from build123d import *

# Parameters (mm, degrees)
EXTRUDE_1_DEPTH        = 900
EXTRUDE_1_2_DEPTH      = 900
EXTRUDE_2_DEPTH        = 1720
EXTRUDE_2_2_DEPTH      = 1720
SKETCH_4_W             = 50
SKETCH_4_H             = 60
CUT_EXTRUDE_1_DEPTH    = 10
SKETCH_5_W             = 50
SKETCH_5_H             = 60
CUT_EXTRUDE_2_DEPTH    = 10
SKETCH_6_W             = 60
SKETCH_6_H             = 25
EXTRUDE_3_DEPTH        = 1720
PATTERN_LINEAR_1_COUNT = 2
PATTERN_LINEAR_1_PITCH = 600
SKETCH_7_W             = 25
SKETCH_7_H             = 60
EXTRUDE_4_DEPTH        = 1729
PATTERN_LINEAR_2_COUNT = 5
PATTERN_LINEAR_2_PITCH = 300


with BuildPart() as part:
    # Sketch 1 → Extrude 1 (new, symmetric)
    with BuildSketch(Plane(origin=(0, 0, 0), x_dir=(0, 0, -1), z_dir=(1, 0, 0))):
        Polygon((30, 0), (-30, 0), (-30, 40), (-10, 40), (-10, 50), (10, 50), (10, 40), (30, 40), align=None)
    extrude(amount=EXTRUDE_1_DEPTH, both=True)

    # Sketch 5 → Cut-Extrude 2 (cut)
    with BuildSketch(Plane(origin=(0, 40, 0), x_dir=(1, 0, 0), z_dir=(0, 1, 0))):
        with Locations((-875, 0)):
            Rectangle(SKETCH_5_W, SKETCH_5_H)
        with Locations((875, 0)):
            Rectangle(SKETCH_5_W, SKETCH_5_H)
    extrude(amount=CUT_EXTRUDE_2_DEPTH, mode=Mode.SUBTRACT)



with BuildPart() as body_2:
    # Sketch 1 → Extrude 1 2 (new, symmetric)
    with BuildSketch(Plane(origin=(0, 0, 0), x_dir=(0, 0, -1), z_dir=(1, 0, 0))):
        Polygon((30, 1800), (30, 1760), (10, 1760), (10, 1750), (-10, 1750), (-10, 1760), (-30, 1760), (-30, 1800), align=None)
    extrude(amount=EXTRUDE_1_2_DEPTH, both=True)

    # Sketch 4 → Cut-Extrude 1 (cut)
    with BuildSketch(Plane.XZ.offset(-1760)):
        with Locations((-875, 0)):
            Rectangle(SKETCH_4_W, SKETCH_4_H)
        with Locations((875, 0)):
            Rectangle(SKETCH_4_W, SKETCH_4_H)
    extrude(amount=CUT_EXTRUDE_1_DEPTH, mode=Mode.SUBTRACT)


with BuildPart() as body_3:
    # Sketch 3 → Extrude 2 (new body)
    with BuildSketch(Plane.XZ.offset(-1760)):
        Polygon((-900, -30), (-900, 30), (-860, 30), (-860, 10), (-850, 10), (-850, -10), (-860, -10), (-860, -30), align=None)
    extrude(amount=EXTRUDE_2_DEPTH)



with BuildPart() as body_4:
    # Sketch 3 → Extrude 2 2 (new body)
    with BuildSketch(Plane.XZ.offset(-1760)):
        Polygon((860, -30), (900, -30), (900, 30), (860, 30), (860, 10), (850, 10), (850, -10), (860, -10), align=None)
    extrude(amount=EXTRUDE_2_2_DEPTH)


with BuildPart() as body_3_1:
    add(body_3.part)

    add(body_4.part)  # Extrude 3 merges body 4
    # Sketch 6 → Extrude 3 (add)
    with BuildSketch(Plane.ZY.offset(-860)):
        with Locations((0, 1200)):
            Rectangle(SKETCH_6_W, SKETCH_6_H)
    extrude_3 = extrude(amount=EXTRUDE_3_DEPTH)

    # Pattern Linear 1: Extrude 3 ×2
    with Locations(*[(0, -i * PATTERN_LINEAR_1_PITCH, 0) for i in range(1, PATTERN_LINEAR_1_COUNT)]):
        add(extrude_3)


with BuildPart() as part_1:
    add(part.part)

    add(body_2.part)  # Extrude 4 merges body 2

    add(body_3_1.part)  # Extrude 4 merges body 3
    # Sketch 7 → Extrude 4 (add)
    with BuildSketch(Plane.XZ.offset(-1760)):
        with Locations((-600, 0)):
            Rectangle(SKETCH_7_W, SKETCH_7_H)
    extrude_4 = extrude(amount=EXTRUDE_4_DEPTH)

    # Pattern Linear 2: Extrude 4 ×5
    with Locations(*[(i * PATTERN_LINEAR_2_PITCH, 0, 0) for i in range(1, PATTERN_LINEAR_2_COUNT)]):
        add(extrude_4)


solid = part_1.part
The model under review builds one solid part; all positions refer to its coordinate system, in mm. A direction names the side the tool comes from. Round coordinates to 2 decimals unless told otherwise and drop trailing zeros. Loops run counter-clockwise (first coordinate to the right, second up) from the corner with the lowest first, then second, coordinate; pieces in that order, holes last. Notation, with made-up numbers: (57.25, 8) -> (62.25, 8) arc R22 cw to (62.25, 34) -> close; hole circle Ø8 at (25.5, -11). An arc over 180 degrees is marked (long way). One line per question, with ' | ' between items. Start each with the question number.
Item 1: Wall thickness on line 1 along Y through (x, z) = (348, 5); line 2 along Y through (x, z) = (-767.5, 18.5): over which ranges is each line inside the solid? List them lowest first. Write a range as [from, to].
Item 2: Machinability: for faces 1 (the face through (855, 315, -10)), 2 (the face through (-448, 612.5, 0)), 3 (the face through (-855, 315, 10)), which of the approach directions +Z, -Z, +X, -X, +Y, -Y give a long, thin tool a straight path to every point of the face, cutting with its end or side? Answer none if there is none.
Item 3: Add section A-A, the plane x = 192.5. Write out the cut boundary in (y, z).
Item 4: Add section B-B, the plane y = 1316. Count the separate pieces of the cut face and the enclosed holes in it, then the cut area to 3 significant figures.
Item 5: For pin 1 (3 mm diameter, centred on x = -159.5, y = 42.5, fed in from -Z), flat-tipped, find the tip position at first contact; note if it passes through.
Item 6: Draft analysis for pull direction Y (two halves, no side actions). For faces 4 (the face through (13, 0, 0)), 5 (the face through (152, 587.5, 0)), state which applies: +Y half, -Y half, draft (parallel to the pull), parting line (faces both ways), or undercut.
Return value:
1) line 1: y = [0, 50], [587.5, 612.5], [1187.5, 1212.5], [1750, 1800] | line 2: y = [0, 40], [587.5, 612.5], [1187.5, 1212.5], [1760, 1800]
2) face 1: -Z | face 2: +Z, -Z | face 3: +Z
3) outline: (0, -30) -> (40, -30) -> (40, -10) -> (50, -10) -> (50, 10) -> (40, 10) -> (40, 30) -> (0, 30) -> close; (587.5, -30) -> (612.5, -30) -> (612.5, 30) -> (587.5, 30) -> close; (1187.5, -30) -> (1212.5, -30) -> (1212.5, 30) -> (1187.5, 30) -> close; (1750, -10) -> (1760, -10) -> (1760, -30) -> (1800, -30) -> (1800, 30) -> (1760, 30) -> (1760, 10) -> (1750, 10) -> close
4) separate pieces: 7 | enclosed holes: 0 | area: 12,700 mm2
5) pin 1: stops at z = -10
6) face 4: -Y half | face 5: undercut
